Part model, mm, in its own coordinate system. Face numbers are marked on the shaded views. A direction names the side the tool comes from. Round coordinates to 2 decimals unless told otherwise and drop trailing zeros. Answer as a JSON object with one key per item and string values.
```python
from build123d import *

# Parameters (mm, degrees)
F1_DEPTH      = 12.5
F1_DEPTH_BACK = 12.5
F0_R          = 2.8070950027
F2_DEPTH      = 10
F2_DEPTH_BACK = 10
F3_DEPTH      = 10
F3_DEPTH_BACK = 10
F4_SIZE       = 2


with BuildPart() as f1:
    # F0 (on Top) → F1 (new body, two sides)
    with BuildSketch(Plane.XY) as f1_sk:
        with BuildLine():
            Line((23.6399736516, 10.5625083831), (23.6399736516, 22.7182886664))
            ThreePointArc((23.6399736516, 22.7182886664), (-13.6170982298, 29.8252180206), (-32.6508275376, -2.9820220135))
            Line((-32.6508275376, -2.9820220135), (4.9928135947, -10.4654852259))
            ThreePointArc((4.9928135947, -10.4654852259), (5.9769233021, -9.8277169412), (7.0685930008, -9.3993741227))
            Line((7.0685930008, -9.3993741227), (23.6399736516, -4.7530159354))
            Line((23.6399736516, -4.7530159354), (23.6399736516, 5.5410303175))
            Line((23.6399736516, 5.5410303175), (14.6979210516, 5.5410303175))
            add(Edge.make_bspline(
                [(14.6979210516, 5.5410303175), (13.8268778101, 6.4642787911), (12.7868333876, 7.4491397486), (13.3415861205, 10.1059010181), (14.6979210516, 10.5625083831)],
                knots=[0, 0, 0, 0, 0.4816059779, 1, 1, 1, 1], degree=3))
            Line((14.6979210516, 10.5625083831), (23.6399736516, 10.5625083831))
        make_face()
    extrude(amount=F1_DEPTH)
    extrude(f1_sk.sketch, amount=-F1_DEPTH_BACK)



with BuildPart() as f1b:
    # F0 (on Top) → F1, piece 2 (new body, two sides)
    with BuildSketch(Plane.XY) as f1_2_sk:
        with BuildLine():
            ThreePointArc((-32.2322682046, -6.0041552748), (-9.3966720268, -31.4113283546), (23.6399736516, -22.7182886664))
            Line((23.6399736516, -22.7182886664), (23.6399736516, -15.8816520533))
            Line((23.6399736516, -15.8816520533), (14.4234997289, -15.8816520533))
            ThreePointArc((14.4234997289, -15.8816520533), (7.2168926216, -20.6875953396), (3.1520300545, -13.0384666845))
            Line((3.1520300545, -13.0384666845), (-32.2322682046, -6.0041552748))
        make_face()
        with Locations((-9.9038304761, -20.5706935376)):
            Circle(F0_R, mode=Mode.SUBTRACT)
    extrude(amount=F1_DEPTH)
    extrude(f1_2_sk.sketch, amount=-F1_DEPTH_BACK)


with BuildPart() as f1_1:
    add(f1.part)

    add(f1b.part)  # F2 merges F1b
    # F0 (on Top) → F2 (join, two sides)
    with BuildSketch(Plane.XY) as f2_sk:
        with BuildLine():
            Line((4.9928135947, -10.4654852259), (-32.6508275376, -2.9820220135))
            ThreePointArc((-32.6508275376, -2.9820220135), (-32.4767201336, -4.4979599312), (-32.2322682046, -6.0041552748))
            Line((-32.2322682046, -6.0041552748), (3.1520300545, -13.0384666845))
            ThreePointArc((3.1520300545, -13.0384666845), (3.8949132368, -11.6249813025), (4.9928135947, -10.4654852259))
        make_face()
    extrude(amount=F2_DEPTH)
    extrude(f2_sk.sketch, amount=-F2_DEPTH_BACK)

    # F0 (on Top) → F3 (join, two sides)
    with BuildSketch(Plane.XY) as f3_sk:
        with Locations((-9.9038304761, -20.5706935376)):
            Circle(F0_R)
    extrude(amount=F3_DEPTH)
    extrude(f3_sk.sketch, amount=-F3_DEPTH_BACK)

    # F4
    f4_edges = [f1_1.edges().sort_by_distance(p)[0] for p in [
        (-13.617098, 29.825218, 12.5),
        (-9.396672, -31.411328, 12.5),
        (-13.617098, 29.825218, -12.5),
        (-9.396672, -31.411328, -12.5),
    ]]
    chamfer(f4_edges, length=F4_SIZE)


solid = f1_1.part
```
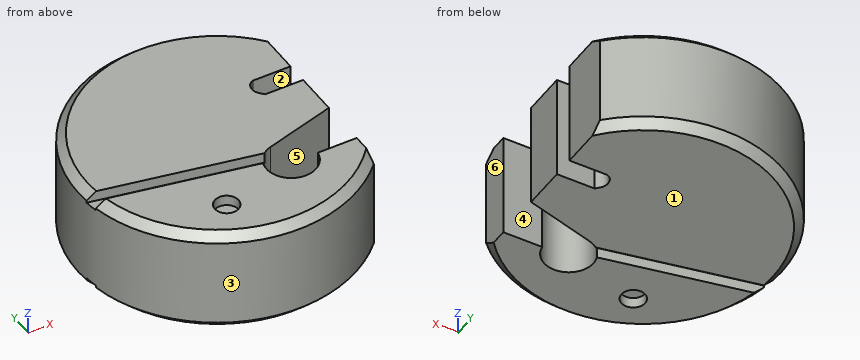
Item 1: Tool access for the marked faces 5 and 6: list every direction of +Z, -Z, +X, -X, +Y, -Y with a clear straight run to the whole face (end or side of a thin tool).
Taken from the geometry:
{"face 5": "+Z, -Z, +X", "face 6": "+Z, -Z, +X, +Y, -Y"}
Item 2: Drop flat-ended pins along their axis: P1, Ø1.7, axis at x = -10, y = -22, coming from the +Z side; P2, Ø1, axis at x = -5.5, z = -10, coming from the -Y side; P3, Ø6, axis at y = 16, z = -9, coming from the -X side; P4, Ø9, axis at x = -9.9, y = -20.57, coming from the +Z side. Give the stop position or say it passes through.
Taken from the geometry:
{"P1": "z = 10", "P2": "y = -32.4", "P3": "x = -30.1", "P4": "z = 12.5"}
Item 3: Two-plate mould, pull along Y, no slides. Class the marked faces 1, 2, 3 and 4: pulls with the +Y half, pulls with the -Y half, needs draft (parallel to the pull), parting line crosses it, or undercut.
Taken from the geometry:
{"face 1": "needs draft", "face 2": "undercut", "face 3": "parting line crosses it", "face 4": "undercut"}
Item 4: Probe L1, parallel to Y at x = 14.5, z = -8.5; L2, parallel to Y at x = 1, z = 2.25; L3, parallel to Y at x = -10, z = -10.75. List the from-to ranges inside material, lowest first. Write a range as from..to.
Taken from the geometry:
{"L1": "-29.41..-15.88, -7.32..5.75, 10.49..29.41", "L2": "-32.77..32.77", "L3": "-30.96..-23.38, -17.77..-10.42, -7.48..30.96"}
